```python
from build123d import *

# Parameters (mm, degrees)
BOSS_EXTRUDE1_DEPTH      = 3.175
BOSS_EXTRUDE1_DEPTH_BACK = 3.175
SKETCH1_R                = 14.2875
SKETCH1_R_2              = 3.429
CUT_EXTRUDE1_DEPTH       = 4.175
CUT_EXTRUDE1_DEPTH_BACK  = 4.175


with BuildPart() as part:
    # Sketch2 → Boss-Extrude1 (new body, two sides)
    with BuildSketch(Plane(origin=(0, 0, 0), x_dir=(0, 0, -1), z_dir=(1, 0, 0))) as boss_extrude1_sk:
        with BuildLine():
            Line((-80.077770294, 30.595392043), (-80.077770294, 58.247946829))
            ThreePointArc((-80.077770294, 58.247946829), (-69.442421386, 66.593204099), (-56.188647306, 69.256179485))
            ThreePointArc((-56.188647306, 69.256179485), (-46.886526626, 70.672129884), (-38.738117997, 75.377212399))
            ThreePointArc((-38.738117997, 75.377212399), (5.090213079, 124.221234623), (34.945098816, 182.662204067))
            ThreePointArc((34.945098816, 182.662204067), (34.521299637, 189.805593755), (29.082706129, 194.456327313))
            Line((29.082706129, 194.456327313), (28.518829965, 194.634116785))
            ThreePointArc((28.518829965, 194.634116785), (23.157656737, 199.132675263), (22.547695998, 206.104558413))
            Line((22.547695998, 206.104558413), (33.54631132, 240.987709604))
            ThreePointArc((33.54631132, 240.987709604), (39.794309207, 248.433783532), (49.477480248, 249.280951225))
            Line((49.477480248, 249.280951225), (122.150711895, 226.367169303))
            ThreePointArc((122.150711895, 226.367169303), (139.389035794, 211.778713703), (141.073716499, 189.25884029))
            ThreePointArc((141.073716499, 189.25884029), (140.738510253, 182.410880382), (144.011829817, 176.386571529))
            Line((144.011829817, 176.386571529), (162.117995595, 161.015451766))
            ThreePointArc((162.117995595, 161.015451766), (165.394045644, 157.419573471), (167.652590835, 153.111230605))
            Line((167.652590835, 153.111230605), (176.079337299, 130.366637638))
            ThreePointArc((176.079337299, 130.366637638), (176.293542275, 122.170313769), (171.454830285, 115.551214511))
            ThreePointArc((171.454830285, 115.551214511), (158.356459409, 107.777887749), (144.240443192, 102.05687257))
            ThreePointArc((144.240443192, 102.05687257), (138.406050553, 98.151824286), (135.537778495, 91.743817189))
            ThreePointArc((135.537778495, 91.743817189), (122.733798507, 80.828311157), (110.332946369, 92.199724514))
            Line((110.332946369, 92.199724514), (110.287974786, 92.199724514))
            Line((110.287974786, 92.199724514), (110.287974786, 106.169724514))
            ThreePointArc((110.287974786, 106.169724514), (108.428102847, 110.659852575), (103.937974786, 112.519724514))
            Line((103.937974786, 112.519724514), (94.944067794, 112.519724514))
            ThreePointArc((94.944067794, 112.519724514), (90.453939734, 110.659852575), (88.594067794, 106.169724514))
            Line((88.594067794, 106.169724514), (88.594067794, 92.199724514))
            Line((88.594067794, 92.199724514), (88.594067794, 89.813112686))
            ThreePointArc((88.594067794, 89.813112686), (81.258269009, 80.137892516), (69.150347517, 81.044571224))
            ThreePointArc((69.150347517, 81.044571224), (63.214959672, 82.045828247), (58.4047538, 78.427366702))
            Line((58.4047538, 78.427366702), (40.912383352, 47.86429176))
            ThreePointArc((40.912383352, 47.86429176), (40.172936643, 42.0792631), (43.740701856, 37.465762324))
            Line((43.740701856, 37.465762324), (51.225250159, 33.182080404))
            ThreePointArc((51.225250159, 33.182080404), (56.134461156, 16.205485457), (39.322849283, 10.758024134))
            ThreePointArc((39.322849283, 10.758024134), (34.662129764, 11.127507824), (31.011761812, 8.206268627))
            Line((31.011761812, 8.206268627), (19.850909717, -11.336709549))
            ThreePointArc((19.850909717, -11.336709549), (11.476550434, -19.770391755), (0, -22.86))
            Line((0, -22.86), (-30.48, -22.86))
            ThreePointArc((-30.48, -22.86), (-35.868153673, -20.628153673), (-38.1, -15.24))
            Line((-38.1, -15.24), (-38.1, 9.584314079))
            ThreePointArc((-38.1, 9.584314079), (-40.331846327, 14.972467752), (-45.72, 17.204314079))
            Line((-45.72, 17.204314079), (-57.217770294, 17.204314079))
            ThreePointArc((-57.217770294, 17.204314079), (-65.965913557, 18.944427966), (-73.382231312, 23.899853061))
            Line((-73.382231312, 23.899853061), (-80.077770294, 30.595392043))
        make_face()
    extrude(amount=BOSS_EXTRUDE1_DEPTH)
    extrude(boss_extrude1_sk.sketch, amount=-BOSS_EXTRUDE1_DEPTH_BACK)

    # Sketch1 → Cut-Extrude1 (cut, two sides)
    with BuildSketch(Plane(origin=(0, 0, 0), x_dir=(0, 0, -1), z_dir=(1, 0, 0))) as cut_extrude1_sk:
        Circle(SKETCH1_R)
        with Locations((-57.217770294, 40.064314079)):
            Circle(SKETCH1_R)
        with Locations((113.367095492, 198.509097171)):
            Circle(SKETCH1_R)
        with Locations((-29.436520294, 42.726234079)):
            Circle(SKETCH1_R_2)
        with Locations((21.363479706, 93.526234079)):
            Circle(SKETCH1_R_2)
        with Locations((122.963479706, 93.526234079)):
            Circle(SKETCH1_R_2)
        with Locations((98.744155059, 176.904777846)):
            Circle(SKETCH1_R_2)
        with Locations((85.377782271, 134.512059385)):
            Circle(SKETCH1_R_2)
        with BuildLine():
            Line((30.555516965, 28.585224085), (30.360175827, 28.148630754))
            ThreePointArc((30.360175827, 28.148630754), (30.289083082, 25.61101973), (32.033174884, 23.766387604))
            Line((32.033174884, 23.766387604), (43.366777865, 18.695492686))
            ThreePointArc((43.366777865, 18.695492686), (45.904388889, 18.624399941), (47.749021015, 20.368491743))
            Line((47.749021015, 20.368491743), (47.944362153, 20.805085073))
            ThreePointArc((47.944362153, 20.805085073), (48.015454897, 23.342696098), (46.271363096, 25.187328223))
            Line((46.271363096, 25.187328223), (34.937760115, 30.258223141))
            ThreePointArc((34.937760115, 30.258223141), (32.40014909, 30.329315886), (30.555516965, 28.585224085))
        make_face()
        with BuildLine():
            Line((36.134107155, 219.131995286), (45.218261111, 216.267772546))
            ThreePointArc((45.218261111, 216.267772546), (49.67898841, 218.5898802), (47.356880757, 223.0506075))
            Line((47.356880757, 223.0506075), (38.272726801, 225.91483024))
            ThreePointArc((38.272726801, 225.91483024), (33.811999501, 223.592722586), (36.134107155, 219.131995286))
        make_face()
        with BuildLine():
            Line((61.67607301, 98.140604836), (61.480731873, 97.704011505))
            ThreePointArc((61.480731873, 97.704011505), (61.409639128, 95.166400481), (63.153730929, 93.321768355))
            Line((63.153730929, 93.321768355), (74.487333911, 88.250873437))
            ThreePointArc((74.487333911, 88.250873437), (77.024944935, 88.179780692), (78.86957706, 89.923872494))
            Line((78.86957706, 89.923872494), (79.064918198, 90.360465824))
            ThreePointArc((79.064918198, 90.360465824), (79.136010943, 92.898076849), (77.391919142, 94.742708974))
            Line((77.391919142, 94.742708974), (66.05831616, 99.813603892))
            ThreePointArc((66.05831616, 99.813603892), (63.520705136, 99.884696637), (61.67607301, 98.140604836))
        make_face()
        with BuildLine():
            Line((70.728471243, 123.847620068), (37.643621714, 142.742135984))
            ThreePointArc((37.643621714, 142.742135984), (36.366491689, 147.420278874), (41.044634579, 148.697408899))
            Line((41.044634579, 148.697408899), (74.129484108, 129.802892984))
            ThreePointArc((74.129484108, 129.802892984), (75.406614133, 125.124750094), (70.728471243, 123.847620068))
        make_face()
        with BuildLine():
            ThreePointArc((118.126670603, 144.106904708), (110.04531429, 134.475919289), (119.676299709, 126.394562976))
            ThreePointArc((119.676299709, 126.394562976), (138.125933667, 130.484748353), (154.888293719, 139.210680685))
            ThreePointArc((154.888293719, 139.210680685), (157.071460874, 151.592036878), (144.690104681, 153.775204033))
            ThreePointArc((144.690104681, 153.775204033), (132.044815519, 147.19248315), (118.126670603, 144.106904708))
        make_face()
        with BuildLine():
            ThreePointArc((116.483795739, 162.885050332), (114.059388845, 159.995754706), (116.948684471, 157.571347812))
            ThreePointArc((116.948684471, 157.571347812), (127.422113984, 159.893251235), (136.937717213, 164.846760742))
            ThreePointArc((136.937717213, 164.846760742), (137.59266736, 168.5611676), (133.878260502, 169.216117746))
            ThreePointArc((133.878260502, 169.216117746), (125.597778539, 164.905571674), (116.483795739, 162.885050332))
        make_face()
        with BuildLine():
            ThreePointArc((120.854285842, 112.930119872), (118.429878948, 110.040824247), (121.319174574, 107.616417353))
            ThreePointArc((121.319174574, 107.616417353), (144.572970647, 112.771659829), (165.700137899, 123.769766971))
            ThreePointArc((165.700137899, 123.769766971), (166.355088045, 127.484173829), (162.640681187, 128.139123976))
            ThreePointArc((162.640681187, 128.139123976), (142.748635202, 117.783980268), (120.854285842, 112.930119872))
        make_face()
    extrude(amount=CUT_EXTRUDE1_DEPTH, mode=Mode.SUBTRACT)
    extrude(cut_extrude1_sk.sketch, amount=-CUT_EXTRUDE1_DEPTH_BACK, mode=Mode.SUBTRACT)


solid = part.part
```
The model under review builds one solid part; all positions refer to its coordinate system, in mm. A direction names the side the tool comes from. Give positions to 0.01 mm unless a question says otherwise; leave off trailing zeros. Write each loop counter-clockwise with the first axis right and the second up, starting at its lowest first coordinate (ties: lowest second). Pieces come first, ordered by that corner, then holes.
(1) Consider section B-B, the plane x = 0.75. Give the number of separate pieces and of enclosed holes in the cut face, and give its area (3 significant figures).
(2) To check wall thickness, follow L1, parallel to Z at x = -2, y = 142; L2, parallel to Y at x = 2.25, z = -39.5; L3, parallel to Y at x = -0.75, z = -132. State the ranges of each line that lie inside material, in increasing order.
(3) The part is to be moulded in two halves that separate along Y. For faces 1 (the flat face through (0.044, 90.822, -68.741)), 2 (the flat face through (0, 99, -110.288)), 3 (the cylindrical face through (0.044, -20.687, 35.809)), 4 (the cylindrical face through (0.04, 112.66, -144.26)), say which applies: released by +Y, released by -Y, zero draft, split by the parting line, or undercut.
(4) For P1, Ø3, axis at x = -1, z = -100, coming from the -Y side; P2, Ø9, axis at y = 93.53, z = -21.36, coming from the -X side (3 decimals); P3, Ø2, axis at x = 1, z = 54, coming from the +Y side; P4, Ø4, axis at y = 93.53, z = -122.96, coming from the +X side, all flat-tipped, find the tip position at first contact; note any pin that passes through.
(5) Tool access review of faces 5 (the cylindrical face through (0.044, 110.709, -90.504)), 6 (the cylindrical face through (0.044, 182.506, -140.717)), 7 (the cylindrical face through (0.04, 164.95, -125.72)): name each direction out of +Z, -Z, +X, -X, +Y, -Y from which nothing blocks a thin tool from reaching the whole face with its end or side.
(6) Consider section A-A, the plane y = 0. Give the boundary of the cut face in (x, z) (1 decimal).
Returned:
1. separate pieces: 1
1. enclosed holes: 15
1. area: 27,000 mm2
2. L1: z = -171.77 to -157.46, -113.12 to -52.77, -38.94 to -16.25
2. L2: y = 10.67 to 20.43, 28.22 to 141.68, 149.15 to 218.07, 225.53 to 248.28
2. L3: y = 84.6 to 109.19, 114.65 to 128.56, 147.18 to 161.88, 167.99 to 221
3. face 1: undercut
3. face 2: zero draft
3. face 3: released by -Y
3. face 4: undercut
4. P1: stops at y = 112.52
4. P2: stops at x = -3.175
4. P3: stops at y = 69.34
4. P4: passes through
5. face 5: +X, -X, -Y
5. face 6: -Z, +X, -X
5. face 7: +X, -X
6. outline: (-3.2, -26.3) - (3.2, -26.3) - (3.2, -14.3) - (-3.2, -14.3) - close; (-3.2, 14.3) - (3.2, 14.3) - (3.2, 38.1) - (-3.2, 38.1) - close
